Model file for the job. Use its own axes, mm. Give positions to 0.01 mm unless a question says otherwise; leave off trailing zeros. Order: outer loops, then holes, each group sorted by start corner. A loop starts at its lowest first (then second) coordinate and runs counter-clockwise, first axis right, second up. Notation, with made-up numbers: (61.25, -16) - (110.25, -16) arc R18 cw to (110.25, 14) - close; hole circle Ø7 at (22.25, 15). An arc over 180 degrees is marked (long way). Use CSV: the item, a comma, the result in double quotes. Start each with the question number.
(1) Band-saw the part on A-A, the plane y = -7. Give the cut face in (x, z).
(2) Band-saw the part on B-B, the plane z = 2. Count the separate pieces of the cut face and the enclosed holes in it, then the cut area to 3 significant figures.
(3) Probe L1, parallel to X at y = -6, z = 2.35; L2, parallel to X at y = -3.5, z = 1.25; L3, parallel to Y at x = -34, z = 2.55. List the from-to ranges inside material, lowest first.
(4) Drop flat-ended pins along their axis: pin 1 Ø5 at (x, y) = (38.5, 7.5) entering from -Z; pin 2 Ø2 at (x, z) = (20.5, 1.5) entering from -Y. Give the stop position or say it passes through.
from build123d import *

# Parameters (mm, degrees)
SKETCH_1_R      = 1.5
EXTRUDE_1_DEPTH = 5
CHAMFER_1_SIZE  = 5


with BuildPart() as part:
    # 草图1 → 凸台-拉伸1 (new body)
    with BuildSketch(Plane.XY):
        Polygon((-82.356314269, -20), (-22.25, -20), (-22.25, -5), (-23.65, -5), (-23.65, -1.5), (-22.25, -1.5), (-22.25, 5), (-17.75, 5), (-17.75, -1.5), (-16.35, -1.5), (-16.35, -5), (-17.75, -5), (-17.75, -20), (17.75, -20), (17.75, -5), (16.35, -5), (16.35, -1.5), (17.75, -1.5), (17.75, 5), (22.25, 5), (22.25, -1.5), (23.65, -1.5), (23.65, -5), (22.25, -5), (22.25, -20), (82.356314269, -20), (82.356314269, 20), (-82.356314269, 20), align=None)
        with Locations((-64.67246571, 14.67246571)):
            Circle(SKETCH_1_R, mode=Mode.SUBTRACT)
        with Locations((-35.32753429, 14.67246571)):
            Circle(SKETCH_1_R, mode=Mode.SUBTRACT)
        with Locations((-64.67246571, -14.67246571)):
            Circle(SKETCH_1_R, mode=Mode.SUBTRACT)
        with Locations((-35.32753429, -14.67246571)):
            Circle(SKETCH_1_R, mode=Mode.SUBTRACT)
        with Locations(Location((64.67246571, 14.67246571, 0), (0, 0, 180))):
            Circle(SKETCH_1_R, mode=Mode.SUBTRACT)
        with Locations(Location((64.67246571, -14.67246571, 0), (0, 0, 180))):
            Circle(SKETCH_1_R, mode=Mode.SUBTRACT)
        with Locations(Location((35.32753429, -14.67246571, 0), (0, 0, 180))):
            Circle(SKETCH_1_R, mode=Mode.SUBTRACT)
        with Locations(Location((35.32753429, 14.67246571, 0), (0, 0, 180))):
            Circle(SKETCH_1_R, mode=Mode.SUBTRACT)
        with Locations((-54.67246571, 14.67246571)):
            Circle(SKETCH_1_R, mode=Mode.SUBTRACT)
        with Locations((-25.32753429, 14.67246571)):
            Circle(SKETCH_1_R, mode=Mode.SUBTRACT)
        with Locations((-54.67246571, -14.67246571)):
            Circle(SKETCH_1_R, mode=Mode.SUBTRACT)
        with Locations((-25.32753429, -14.67246571)):
            Circle(SKETCH_1_R, mode=Mode.SUBTRACT)
        with Locations((-74.67246571, 14.67246571)):
            Circle(SKETCH_1_R, mode=Mode.SUBTRACT)
        with Locations((-45.32753429, 14.67246571)):
            Circle(SKETCH_1_R, mode=Mode.SUBTRACT)
        with Locations((-45.32753429, -14.67246571)):
            Circle(SKETCH_1_R, mode=Mode.SUBTRACT)
        with Locations((-74.67246571, -14.67246571)):
            Circle(SKETCH_1_R, mode=Mode.SUBTRACT)
        with Locations(Location((45.32753429, 14.67246571, 0), (0, 0, 180))):
            Circle(SKETCH_1_R, mode=Mode.SUBTRACT)
        with Locations(Location((45.32753429, -14.67246571, 0), (0, 0, 180))):
            Circle(SKETCH_1_R, mode=Mode.SUBTRACT)
        with Locations(Location((74.67246571, -14.67246571, 0), (0, 0, 180))):
            Circle(SKETCH_1_R, mode=Mode.SUBTRACT)
        with Locations(Location((74.67246571, 14.67246571, 0), (0, 0, 180))):
            Circle(SKETCH_1_R, mode=Mode.SUBTRACT)
        with Locations(Location((25.32753429, 14.67246571, 0), (0, 0, 180))):
            Circle(SKETCH_1_R, mode=Mode.SUBTRACT)
        with Locations(Location((25.32753429, -14.67246571, 0), (0, 0, 180))):
            Circle(SKETCH_1_R, mode=Mode.SUBTRACT)
        with Locations(Location((54.67246571, -14.67246571, 0), (0, 0, 180))):
            Circle(SKETCH_1_R, mode=Mode.SUBTRACT)
        with Locations(Location((54.67246571, 14.67246571, 0), (0, 0, 180))):
            Circle(SKETCH_1_R, mode=Mode.SUBTRACT)
    extrude(amount=EXTRUDE_1_DEPTH)

    # 倒角1
    chamfer_1_edges = [part.edges().sort_by_distance(p)[0] for p in [
        (-82.356314269, 20, 2.5),
        (82.356314269, 20, 2.5),
        (82.356314269, -20, 2.5),
        (-82.356314269, -20, 2.5),
    ]]
    chamfer(chamfer_1_edges, length=CHAMFER_1_SIZE)


solid = part.part
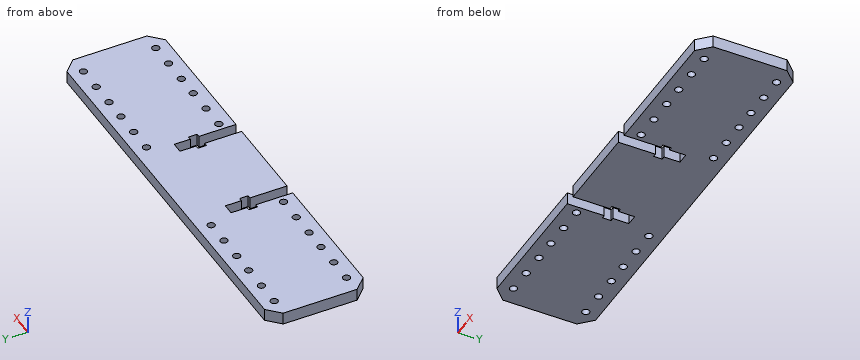
Answer block:
1,outline,"(-82.36, 0) - (-22.25, 0) - (-22.25, 5) - (-82.36, 5) - close; (-17.75, 0) - (17.75, 0) - (17.75, 5) - (-17.75, 5) - close; (22.25, 0) - (82.36, 0) - (82.36, 5) - (22.25, 5) - close"
2,separate pieces,"1"
2,enclosed holes,"24"
2,area,"6,120 mm2"
3,L1,"x = -82.36 to -22.25, -17.75 to 17.75, 22.25 to 82.36"
3,L2,"x = -82.36 to -23.65, -16.35 to 16.35, 23.65 to 82.36"
3,L3,"y = -20 to -15.37, -13.97 to 13.97, 15.37 to 20"
4,pin 1,"stops at z = 0"
4,pin 2,"stops at y = 5"
